Verification items for the finished model (mm, model axes). Round coordinates to 2 decimals unless told otherwise and drop trailing zeros. Order: outer loops, then holes, each group sorted by start corner. A loop starts at its lowest first (then second) coordinate and runs counter-clockwise, first axis right, second up. Notation, with made-up numbers: (88, 54.5) -> (109, 54.5) arc R25 cw to (109, 74.5) -> close; hole circle Ø9 at (38.25, 3). An arc over 180 degrees is marked (long way). Answer in a Markdown table with one row per item. Add a question column.
```python
from build123d import *

# Parameters (mm, degrees)
SKETCH1_W           = 50.8
SKETCH1_H           = 25.4
SKETCH1_W_2         = 45.72
SKETCH1_H_2         = 20.32
BOSS_EXTRUDE1_DEPTH = 127
SKETCH2_R           = 2.54
CUT_EXTRUDE1_DEPTH  = 25.4
SKETCH3_R           = 14.3002
CUT_EXTRUDE2_DEPTH  = 25.4


with BuildPart() as part:
    # Sketch1 → Boss-Extrude1 (new body)
    with BuildSketch(Plane.XY):
        with Locations((-75.184, 73.640461538)):
            Rectangle(SKETCH1_W, SKETCH1_H)
        with Locations((-75.184, 73.640461538)):
            Rectangle(SKETCH1_W_2, SKETCH1_H_2, mode=Mode.SUBTRACT)
    extrude(amount=BOSS_EXTRUDE1_DEPTH)

    # Sketch2 → Cut-Extrude1 (cut)
    with BuildSketch(Plane(origin=(0, 86.340461538, 0), x_dir=(1, 0, 0), z_dir=(0, 1, 0))):
        with Locations(Location((-94.234, -6.35, 0), (0, 0, 180))):
            Circle(SKETCH2_R)
        with Locations(Location((-81.534, -6.35, 0), (0, 0, 180))):
            Circle(SKETCH2_R)
        with Locations(Location((-68.834, -6.35, 0), (0, 0, 180))):
            Circle(SKETCH2_R)
        with Locations(Location((-56.134, -6.35, 0), (0, 0, 180))):
            Circle(SKETCH2_R)
        with Locations(Location((-81.534, -19.05, 0), (0, 0, 180))):
            Circle(SKETCH2_R)
        with Locations(Location((-68.834, -19.05, 0), (0, 0, 180))):
            Circle(SKETCH2_R)
        with Locations(Location((-56.134, -19.05, 0), (0, 0, 180))):
            Circle(SKETCH2_R)
        with Locations(Location((-81.534, -31.75, 0), (0, 0, 180))):
            Circle(SKETCH2_R)
        with Locations(Location((-68.834, -31.75, 0), (0, 0, 180))):
            Circle(SKETCH2_R)
        with Locations(Location((-56.134, -31.75, 0), (0, 0, 180))):
            Circle(SKETCH2_R)
        with Locations(Location((-81.534, -44.45, 0), (0, 0, 180))):
            Circle(SKETCH2_R)
        with Locations(Location((-68.834, -44.45, 0), (0, 0, 180))):
            Circle(SKETCH2_R)
        with Locations(Location((-56.134, -44.45, 0), (0, 0, 180))):
            Circle(SKETCH2_R)
        with Locations(Location((-81.534, -57.15, 0), (0, 0, 180))):
            Circle(SKETCH2_R)
        with Locations(Location((-68.834, -57.15, 0), (0, 0, 180))):
            Circle(SKETCH2_R)
        with Locations(Location((-56.134, -57.15, 0), (0, 0, 180))):
            Circle(SKETCH2_R)
        with Locations(Location((-81.534, -69.85, 0), (0, 0, 180))):
            Circle(SKETCH2_R)
        with Locations(Location((-68.834, -69.85, 0), (0, 0, 180))):
            Circle(SKETCH2_R)
        with Locations(Location((-56.134, -69.85, 0), (0, 0, 180))):
            Circle(SKETCH2_R)
        with Locations(Location((-81.534, -82.55, 0), (0, 0, 180))):
            Circle(SKETCH2_R)
        with Locations(Location((-68.834, -82.55, 0), (0, 0, 180))):
            Circle(SKETCH2_R)
        with Locations(Location((-56.134, -82.55, 0), (0, 0, 180))):
            Circle(SKETCH2_R)
        with Locations(Location((-81.534, -95.25, 0), (0, 0, 180))):
            Circle(SKETCH2_R)
        with Locations(Location((-68.834, -95.25, 0), (0, 0, 180))):
            Circle(SKETCH2_R)
        with Locations(Location((-56.134, -95.25, 0), (0, 0, 180))):
            Circle(SKETCH2_R)
        with Locations(Location((-81.534, -107.95, 0), (0, 0, 180))):
            Circle(SKETCH2_R)
        with Locations(Location((-68.834, -107.95, 0), (0, 0, 180))):
            Circle(SKETCH2_R)
        with Locations(Location((-56.134, -107.95, 0), (0, 0, 180))):
            Circle(SKETCH2_R)
        with Locations(Location((-81.534, -120.65, 0), (0, 0, 180))):
            Circle(SKETCH2_R)
        with Locations(Location((-68.834, -120.65, 0), (0, 0, 180))):
            Circle(SKETCH2_R)
        with Locations(Location((-56.134, -120.65, 0), (0, 0, 180))):
            Circle(SKETCH2_R)
        with Locations(Location((-94.234, -19.05, 0), (0, 0, 180))):
            Circle(SKETCH2_R)
        with Locations(Location((-94.234, -31.75, 0), (0, 0, 180))):
            Circle(SKETCH2_R)
        with Locations(Location((-94.234, -44.45, 0), (0, 0, 180))):
            Circle(SKETCH2_R)
        with Locations(Location((-94.234, -57.15, 0), (0, 0, 180))):
            Circle(SKETCH2_R)
        with Locations(Location((-94.234, -69.85, 0), (0, 0, 180))):
            Circle(SKETCH2_R)
        with Locations(Location((-94.234, -82.55, 0), (0, 0, 180))):
            Circle(SKETCH2_R)
        with Locations(Location((-94.234, -95.25, 0), (0, 0, 180))):
            Circle(SKETCH2_R)
        with Locations(Location((-94.234, -107.95, 0), (0, 0, 180))):
            Circle(SKETCH2_R)
        with Locations(Location((-94.234, -120.65, 0), (0, 0, 180))):
            Circle(SKETCH2_R)
    extrude(amount=-CUT_EXTRUDE1_DEPTH, mode=Mode.SUBTRACT)

    # Sketch3 → Cut-Extrude2 (cut)
    with BuildSketch(Plane.XZ.offset(-60.940461538)):
        with Locations(Location((-75.450612599, 64.036338499, 0), (0, 0, 270))):
            Circle(SKETCH3_R)
    extrude(amount=-CUT_EXTRUDE2_DEPTH, mode=Mode.SUBTRACT)


solid = part.part
```
1) Cross-section at D-D, the plane x = -64. Record the boundary of the cut face in (y, z), and give its area (3 significant figures).
2) Draft check along Z on faces 1 (the face through (-49.784, 73, 63)), 2 (the face through (-70.2, 85.09, 97.39)). Enter one of: +Z half, -Z half, draft (parallel to the pull), parting line (faces both ways), or undercut.
3) Cross-section at C-C, the plane z = 58.5. Give the number of separate pieces and of enclosed holes in the cut face, and give its area (3 significant figures).
4) Thickness scan on L1, parallel to X at y = 64.75, z = 52; L2, parallel to Y at x = -69, z = 22; L3, parallel to X at y = 84.5, z = 45. Record the ranges inside material, lowest first. Write a range as [from, to].
5) Cross-section at B-B, the plane x = -88. Record the boundary of the cut face in (y, z), and give its area (4 significant figures).
6) Depth check by flat-ended pin: P1, Ø12, axis at x = -67.5, y = 65.5, coming from the +Z side. Enter the tip coordinate at first touch or a pass-through.
7) Cross-section at A-A, the plane y = 67.25. Record the boundary of the cut face in (x, z), and give its area (3 significant figures).
Results below:
| question | item | result |
|---|---|---|
| 1 | outline | (60.94, 0) -> (63.48, 0) -> (63.48, 55.47) -> (60.94, 55.47) -> close; (60.94, 72.6) -> (63.48, 72.6) -> (63.48, 127) -> (60.94, 127) -> close; (83.8, 0) -> (86.34, 0) -> (86.34, 55.47) -> (83.8, 55.47) -> close; (83.8, 72.6) -> (86.34, 72.6) -> (86.34, 127) -> (83.8, 127) -> close |
| 1 | area | 558 mm² |
| 2 | face 1 | draft |
| 2 | face 2 | undercut |
| 3 | separate pieces | 6 |
| 3 | enclosed holes | 0 |
| 3 | area | 184 mm² |
| 4 | L1 | [-100.58, -98.04], [-52.32, -49.78] |
| 4 | L2 | [60.94, 63.48], [83.8, 86.34] |
| 4 | L3 | [-100.58, -96.71], [-91.75, -84.01], [-79.05, -71.31], [-66.35, -58.61], [-53.65, -49.78] |
| 5 | outline | (60.94, 0) -> (63.48, 0) -> (63.48, 57.18) -> (60.94, 57.18) -> close; (60.94, 70.89) -> (63.48, 70.89) -> (63.48, 127) -> (60.94, 127) -> close; (83.8, 0) -> (86.34, 0) -> (86.34, 57.18) -> (83.8, 57.18) -> close; (83.8, 70.89) -> (86.34, 70.89) -> (86.34, 127) -> (83.8, 127) -> close |
| 5 | area | 575.5 mm² |
| 6 | P1 | z = 127 |
| 7 | outline | (-100.58, 0) -> (-98.04, 0) -> (-98.04, 127) -> (-100.58, 127) -> close; (-52.32, 0) -> (-49.78, 0) -> (-49.78, 127) -> (-52.32, 127) -> close |
| 7 | area | 645 mm² |
